Autodesk Inventor part; units mm, degrees
ref_plane "YZ Plane" through (0, 0, 0) normal (1, 0, 0) x (0, 1, 0)
ref_plane "XZ Plane" through (0, 0, 0) normal (0, 1, 0) x (-1, 0, 0)
ref_plane "XY Plane" through (0, 0, 0) normal (0, 0, 1) x (1, 0, 0)
sketch "スケッチ1" plane through (0, 0, 0) normal (0, 0, 1) x (1, 0, 0)
  circle A0 centre (0, 0) radius 42.25
  circle A1 centre (0, 0) radius 53.25
  circle A2 centre (0, 0) radius 49.25
  circle A3 centre (0, 0) radius 57.25
  dimension "d0" = 84.5
  dimension "d1" = 11
  dimension "d2" = 4
  dimension "d3" = 4
extrude "押し出し1" add sketch "スケッチ1" along normal blind 2 contours A1 | A3
sketch "スケッチ2" plane through (0, 0, 2) normal (0, 0, 1) x (1, 0, 0)
  line L0 (0, 0) -> (0, 57.25)
  circle A0 centre (0, 0) radius 57.25
  line L1 (0, 0) -> (40.4819, 40.4819)
  circle A1 centre (0, 0) radius 53.25
  circle A2 centre (0, 0) radius 49.25
  point P0 (37.6534, 37.6534)
  point P1 (-37.6534, 37.6534)
  point P2 (-37.6534, -37.6534)
  point P3 (37.6534, -37.6534)
  dimension "d6" = 45
  dimension "d7" = 4
  dimension "d10" = 360
hole "穴1" at (37.6534, 37.6534, 2) at (-37.6534, 37.6534, 2) at (-37.6534, -37.6534, 2) at (37.6534, -37.6534, 2) direction (0, 0, -1) diameter 3.1 end through all
properties part number "base_plate4" material "アルミニウム 6061"
Geometry: final body of the model. Coordinates: model frame, mm. Round coordinates to 2 decimals unless told otherwise and drop trailing zeros. Write each loop counter-clockwise with the first axis right and the second up, starting at its lowest first coordinate (ties: lowest second). Pieces come first, ordered by that corner, then holes.
Item 1: Pin query (flat end, axial travel): P1, Ø6, axis at x = -38.5, y = 29.5, coming from the +Z side; P2, Ø1, axis at y = -15.5, z = 1, coming from the -X side; P3, Ø1, axis at x = 33, z = 1.5, coming from the +Y side. Return the tip coordinate at first contact, or that it passes through.
Item 2: Mould query, pull axis Y, two halves, no side actions, for faces 1 (the face through (-37.722, -36.105, 0.986)), 2 (the face through (-17.2, -46.4, 0)), 3 (the face through (46.976, -14.793, 0.986)), 4 (the face through (-12.41, 55.89, 0.99)). Classes: +Y half, -Y half, draft (parallel to the pull), parting line (faces both ways), or undercut.
Item 3: Section query C-C (z = 1.1). Return loops of the section in (x, y), plus the area to 3 significant figures.
Item 4: Material intervals for L1, parallel to Y at x = 0, z = 1.6; L2, parallel to X at y = 1, z = 0.3; L3, parallel to Y at x = 27.5, z = 1.1, sorted ascending.
Item 5: Section query A-A (x = 0). Return loops of the section in (y, z).
Completed:
1. P1: stops at z = 2
1. P2: stops at x = -55.25
1. P3: stops at y = 47.13
2. face 1: undercut
2. face 2: draft
2. face 3: undercut
2. face 4: parting line
3. outline: circle Ø114.5 at (0, 0); hole circle Ø98.5 at (0, 0); hole circle Ø3.1 at (-37.65, -37.65); hole circle Ø3.1 at (-37.65, 37.65); hole circle Ø3.1 at (37.65, -37.65); hole circle Ø3.1 at (37.65, 37.65)
3. area: 2,650 mm2
4. L1: y = -57.25 to -49.25, 49.25 to 57.25
4. L2: x = -57.24 to -49.24, 49.24 to 57.24
4. L3: y = -50.21 to -40.86, 40.86 to 50.21
5. outline: (-57.25, 0) - (-49.25, 0) - (-49.25, 2) - (-57.25, 2) - close; (49.25, 0) - (57.25, 0) - (57.25, 2) - (49.25, 2) - close
